Geometry check sheet. Reference: the model listing, model coordinates, mm. A direction names the side the tool comes from. Give positions to 0.01 mm unless a question says otherwise; leave off trailing zeros. Order: outer loops, then holes, each group sorted by start corner. A loop starts at its lowest first (then second) coordinate and runs counter-clockwise, first axis right, second up. Notation, with made-up numbers: M 8,87 L 57,87 A15 cw 57,91 Z; hole C 38,-1 d9. An arc over 180 degrees is marked long. Use CSV: the item, a comma, the result in double quotes. Start each with the question number.
from build123d import *

# Parameters (mm, degrees)
THICKNESS_T = -3


with BuildPart() as part:
    # Sketch → Revolution (revolve)
    with BuildSketch(Plane.XZ):
        Polygon((0, 0), (-39.5, 0), (-39.5, 88), (-41.5, 88), (-41.5, 105), (0, 105), align=None)
    revolve(axis=Axis((0, 0, 0), (0, 0, 1)))

    # Thickness
    thickness_openings = [part.faces().sort_by_distance(p)[0] for p in [
        (0, 0, 105),
    ]]
    offset(amount=THICKNESS_T, openings=thickness_openings, kind=Kind.INTERSECTION)


solid = part.part
(1) Sectioned sample at A-A on y = 0. Record the cut outline in (x, z), then the cut area to 3 significant figures.
(2) Sectioned sample at C-C on z = 96. Record the cut outline in (x, y), then the cut area to 3 significant figures.
(3) Access from +Z, -Z, +X, -X, +Y, -Y to the whole of each face (thin tool, end or side, straight path). Record for faces 1 (the face through (-39.584, -12.465, 96.619)), 2 (the face through (30.55, 23.43, 98.1)).
(4) Sectioned sample at D-D on z = 74.5. Record the cut outline in (x, y).
(5) Draft check along X on faces 3 (the face through (-1, -1, 3)), 4 (the face through (29.11, -26.7, 44.62)), 5 (the face through (37, 15, 88)). Enter one of: +X half, -X half, draft (parallel to the pull), parting line (faces both ways), or undercut.
(6) Go/stop test with flat-tipped pins: P1, Ø4, axis at y = -1, z = 47, coming from the +X side; P2, Ø1, axis at x = -9.5, y = -5, coming from the +Z side; P3, Ø4, axis at x = 8.5, z = 34, coming from the +Y side. Record where each tip stops, or that it passes through.
(7) Thickness scan on line 1 (X direction, y = 0, z = 100); line 2 (X direction, y = 1, z = 73); line 3 (Y direction, x = 0, z = 69). Record the ranges inside material, lowest first.
Responses:
1,outline,"M -41.5,88 L -39.5,88 L -39.5,0 L 39.5,0 L 39.5,88 L 41.5,88 L 41.5,105 L 38.5,105 L 38.5,91 L 36.5,91 L 36.5,3 L -36.5,3 L -36.5,91 L -38.5,91 L -38.5,105 L -41.5,105 Z"
1,area,"861 mm2"
2,outline,"C 0,0 d83; hole C 0,0 d77"
2,area,"754 mm2"
3,face 1,"+Z, -Z"
3,face 2,"+Z"
4,outline,"C 0,0 d79; hole C 0,0 d73"
5,face 3,"undercut"
5,face 4,"parting line"
5,face 5,"draft"
6,P1,"x = 39.5"
6,P2,"z = 3"
6,P3,"y = 38.96"
7,line 1,"-41.5 to -38.5, 38.5 to 41.5"
7,line 2,"-39.49 to -36.49, 36.49 to 39.49"
7,line 3,"-39.5 to -36.5, 36.5 to 39.5"
